from build123d import *

# Parameters (mm, degrees)
SKETCH1_R           = 4
BOSS_EXTRUDE1_DEPTH = 40
BOSS_EXTRUDE2_DEPTH = 20


with BuildPart() as part:
    # Sketch1 → Boss-Extrude1 (new body)
    with BuildSketch(Plane.XY):
        Circle(SKETCH1_R)
    extrude(amount=BOSS_EXTRUDE1_DEPTH)

    # Sketch2 → Boss-Extrude2 (add)
    with BuildSketch(Plane.XY.offset(40)):
        with BuildLine():
            Line((-2, 13.856406461), (-2, 15))
            Line((-2, 15), (2, 15))
            Line((2, 15), (2, 13.856406461))
            ThreePointArc((2, 13.856406461), (0, -14), (-2, 13.856406461))
        make_face()
    extrude(amount=-BOSS_EXTRUDE2_DEPTH)


solid = part.part
Geometry check sheet. Reference: the model listing, model coordinates, mm. A direction names the side the tool comes from. Give positions to 0.01 mm unless a question says otherwise; leave off trailing zeros. Order: outer loops, then holes, each group sorted by start corner. A loop starts at its lowest first (then second) coordinate and runs counter-clockwise, first axis right, second up. Notation, with made-up numbers: (-14.5, 49) - (-10.5, 49) arc R31 ccw to (-10.5, 84) - close; hole circle Ø4 at (86, 65). An arc over 180 degrees is marked (long way). Answer as a JSON object with one key per item and string values.
(1) Cross-section at B-B (x = 0). Record the cut outline in (y, z), then the cut area to 3 significant figures.
Report:
{"outline": "(-14, 20) - (-4, 20) - (-4, 0) - (4, 0) - (4, 20) - (15, 20) - (15, 40) - (-14, 40) - close", "area": "740 mm^2"}
(2) Cross-section at A-A (y = 0). Record the cut outline in (x, z).
Report:
{"outline": "(-14, 20) - (-4, 20) - (-4, 0) - (4, 0) - (4, 20) - (14, 20) - (14, 40) - (-14, 40) - close"}
(3) Tool access check on faces 1 (the cylindrical face through (0.587, -13.988, 30.14)), 2 (the flat face through (2, 14.4, 30.1)), 3 (the cylindrical face through (-0.867, -3.905, 9.86)), 4 (the flat face through (-2, 14.4, 30.1)). Record the directions out of +Z, -Z, +X, -X, +Y, -Y that give a thin tool (end or side, any length) a straight path to the whole face; none if there is none.
Report:
{"face 1": "+Z, -Z", "face 2": "+Z, -Z, +X, +Y", "face 3": "-Z", "face 4": "+Z, -Z, -X, +Y"}
(4) Depth check by flat-ended pin: pin 1 Ø5 at (y, z) = (6, 9) entering from +X; pin 2 Ø1.5 at (y, z) = (-9, 32.5) entering from -X; pin 3 Ø4 at (y, z) = (-5.5, 13.5) entering from -X; pin 4 Ø1.5 at (y, z) = (7, 17.5) entering from +X. Enter the tip coordinate at first touch or a pass-through.
Report:
{"pin 1": "x = 1.94", "pin 2": "x = -11.31", "pin 3": "x = -1.94", "pin 4": "through"}
(5) Material ranges on line 1 (Z direction, x = -2.75, y = 6.5); line 2 (X direction, y = 3.25, z = 33.5); line 3 (X direction, y = 0.75, z = 37), recorded low to high.
Report:
{"line 1": "20 to 40", "line 2": "-13.62 to 13.62", "line 3": "-13.98 to 13.98"}
(6) Cross-section at C-C (z = 9). Record the cut outline in (x, y), then the cut area to 3 significant figures.
Report:
{"outline": "circle Ø8 at (0, 0)", "area": "50.3 mm^2"}
(7) Cross-section at D-D (z = 33). Record the cut outline in (x, y).
Report:
{"outline": "(-2, 13.86) arc R14 ccw (long way) to (2, 13.86) - (2, 15) - (-2, 15) - close"}
